Model file for the job. Use its own axes, mm. A direction names the side the tool comes from. Give positions to 0.01 mm unless a question says otherwise; leave off trailing zeros. Write each loop counter-clockwise with the first axis right and the second up, starting at its lowest first coordinate (ties: lowest second). Pieces come first, ordered by that corner, then holes.
Autodesk Inventor part; units mm, degrees
ref_plane "YZ Plane" through (0, 0, 0) normal (1, 0, 0) x (0, 1, 0)
ref_plane "XZ Plane" through (0, 0, 0) normal (0, 1, 0) x (-1, 0, 0)
ref_plane "XY Plane" through (0, 0, 0) normal (0, 0, 1) x (1, 0, 0)
sketch "Sketch1" plane through (0, 0, 0) normal (0, 0, 1) x (1, 0, 0)
  circle A0 centre (0, 0) radius 10
  circle A1 centre (0, 0) radius 1
  dimension "d34" = 20
  dimension "d35" = 2
extrude "Extrusion1" add sketch "Sketch1" along normal blind 0.6
sketch "Sketch2" plane through (0, 0, 0.6) normal (0, 0, 1) x (1, 0, 0)
  circle A0 centre (0, 0) radius 10
  circle A1 centre (0, 0) radius 6
  dimension "d8" = 4
extrude "Extrusion2" add sketch "Sketch2" along normal blind 5
fillet "Fillet1" radius 2 3 edges at (-6, 0, 0.6) (-6, 0, 5.6) (-10, 0, 5.6)
sketch "Sketch3" plane through (0, 0, 0) normal (0, 0, -1) x (-1, 0, 0)
  circle A0 centre (0, 0) radius 10
  circle A1 centre (0, -0.75) radius 0.25
  line L0 (-0.2487, -0.7372) -> (-0.25, -0.75)
  line L1 (0, -0.5128) -> (0, -1.0128) construction
  arc A2 (0, -0.5128) -> (-0.2487, -0.7372) centre (0, -0.7628) ccw
  arc A3 (-0.2447, -0.699) -> (0.2447, -0.699) centre (0, -0.75) ccw
  line L2 (0.2487, -0.7372) -> (0.25, -0.75)
  arc A4 (0.2487, -0.7372) -> (0, -0.5128) centre (0, -0.7628) ccw
  point P0 (0, -0.5)
  dimension "d17" = 0.25
sketch "Sketch4" plane through (0, 0, 0) normal (0, 0, -1) x (-1, 0, 0)
  circle A0 centre (0, 0) radius 10
  circle A1 centre (0, 8) radius 2.45
  dimension "d18" = 4.9
  dimension "d19" = 8
extrude "Extrusion4" cut sketch "Sketch4" against normal blind 4 contours A1 A0 | A0 A1 picked at (-0.0666, 8.5101) picked at (0, 10.1407)
pattern_circular "Circular Pattern2" count 3 over 360 about axis through (0, 0, 0) along (0, 0, 1) of "Extrusion4"
sketch "Sketch8" plane through (0, 0, 0) normal (1, 0, 0) x (0, 1, 0)
  line L0 (-3.5716, 0) -> (-3.5716, 3.6)
  line L1 (9.8748, 3.6) -> (-3.5716, 3.6)
  line L2 (9.8748, 3.6) -> (9.8748, 0)
  line L3 (-3.5716, 0) -> (9.8748, 0)
  circle A0 centre (0, 1.3137) radius 0.6099
  point P0 (0, 0)
extrude "Extrusion6" cut sketch "Sketch8" along normal through all both and the other way through all contours A0
properties part number "30_Cube_openSIM_Fouriermask_1"
1. Slice it at C-C, the plane z = 4.5. Write the cut outline in (x, y), and give its area (3 significant figures).
Calculated:
outline: circle Ø19.57 at (0, 0); hole circle Ø12.43 at (0, 0)
area: 180 mm2
2. Which spindle directions (+Z, -Z, +X, -X, +Y, -Y) get a long thin tool onto all of the face, cutting with end or side? Do faces 4 (the flat face through (0, 8, 4)), 5 (the cylindrical face through (-0.217, 0.976, 0.296)), 6 (the cylindrical face through (0, -6, 3)). Say none if no direction does.
Calculated:
face 4: -Z
face 5: +Z, -Z
face 6: +Z
3. Pull direction Y, two halves, no side cores. Call faces 1 (the cylindrical face through (0, -10, 2)), 2 (the cylindrical face through (-8.722, 4.892, 1.775)), 3 (the cylindrical face through (5.16, 3.06, 3.09)): +Y half, -Y half, draft (parallel to the pull), parting line (faces both ways), or undercut.
Calculated:
face 1: -Y half
face 2: parting line
face 3: undercut
4. Slice it at A-A, the plane x = 0. State how many separate pieces and enclosed holes the cut face has, and give its area (3 significant figures).
Calculated:
separate pieces: 3
enclosed holes: 0
area: 32.3 mm2
5. Pin check, flat tips, straight feed: P1, Ø1.8, axis at x = 0, y = 0, coming from the +Z side; P2, Ø3, axis at y = -7.5, z = 4.5, coming from the -X side; P3, Ø4.5, axis at x = -6.93, y = -4, coming from the -Z side; P4, Ø3, axis at y = -6.5, z = 4.5, coming from the -X side. Stop position of each tip, or through.
Calculated:
P1: passes through
P2: stops at x = -7.88
P3: stops at z = 4
P4: stops at x = -8.56
6. Probe probe 1 along X at (y, z) = (8, 1.6); probe 2 along X at (y, z) = (-1, 0.85); probe 3 along Y at (x, z) = (2.75, 0.95). List the from-to ranges inside material, lowest first.
Calculated:
probe 1: x = -6 to -2.45, 2.45 to 6
probe 2: x = -9.95 to -4.87, 4.87 to 9.95
probe 3: y = -9.61 to -4.33, 4.33 to 9.61
